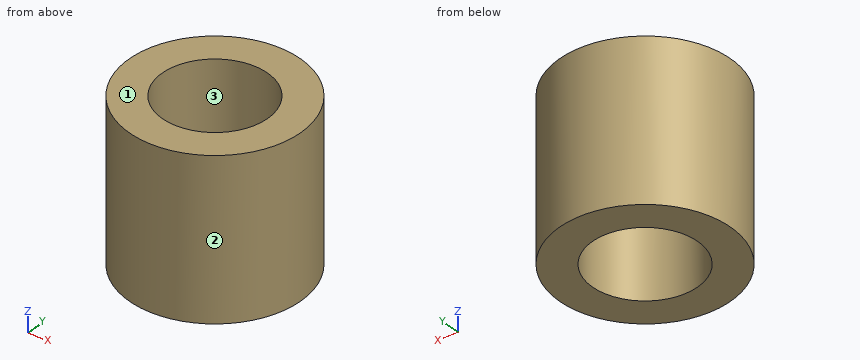
Autodesk Fusion 360 part; units mm, degrees
sketch "Sketch1" plane through (0, 0, 0) normal (0, 0, 1) x (1, 0, 0)
  circle A0 centre (0, 0) radius 2
  circle A1 centre (0, 0) radius 2.75
  dimension "d5" = 4
  dimension "d8" = 5.5
extrude "Extrude2" add sketch "Sketch1" along normal blind 6.6
move_face "OffsetFaces1" offset 0.5 1 faces at (2.7466, -0.1371, 4.4)
extrude "Extrude3" cut 1 faces at (2.8212, 0.1615, 6.6) along direction (0, 0, -1) blind 1.6
extrude "Extrude4" add 1 faces at (2.8212, 0.1615, 5) along direction (0, 0, 1) blind 1
Verification items for the finished model (mm, model axes). Face numbers are marked on the shaded views. Give positions to 0.01 mm unless a question says otherwise; leave off trailing zeros. Order: outer loops, then holes, each group sorted by start corner. A loop starts at its lowest first (then second) coordinate and runs counter-clockwise, first axis right, second up. Notation, with made-up numbers: M 4.25,75 L 47.25,75 A22 cw 47.25,95 Z; hole C 74,-32.5 d9. An arc over 180 degrees is marked long. Use one line per item in the form item = value. Start each with the question number.
Q1. Section check C-C (z = 0.6). Enter the section's corners in (x, y), then the cut area to 3 significant figures.
Q2. Go/stop test with a flat-tipped pin: pin 1 Ø3 at (x, z) = (2, 3.5) entering from +Y. Record where the tip stops, or that it passes through.
Q3. Section check A-A (x = 0). Enter the section's corners in (y, z), then the cut area to 3 significant figures.
Q4. Mould release check, pull along Y, two halves, no side actions. Record for the marked faces 1, 2 and 3: +Y half, -Y half, draft (parallel to the pull), parting line (faces both ways), or undercut.
Q5. Section check D-D (y = 3). Enter the section's corners in (x, z).
Q6. Scan lines: line 1 along Y through (x, z) = (0, 0.8); line 2 along Y through (x, z) = (-1.5, 0.6). Record each from-to range of solid material in increasing order. Write a range as [from, to].
Evaluation:
q1.outline = C 0,0 d6.5; hole C 0,0 d4
q1.area = 20.6 mm2
q2.pin_1 = 3.21
q3.outline = M -3.25,0 L -2,0 L -2,6 L -3.25,6 Z; M 2,0 L 3.25,0 L 3.25,6 L 2,6 Z
q3.area = 15.0 mm2
q4.face_1 = draft
q4.face_2 = parting line
q4.face_3 = undercut
q5.outline = M -1.25,0 L 1.25,0 L 1.25,6 L -1.25,6 Z
q6.line_1 = [-3.25, -2], [2, 3.25]
q6.line_2 = [-2.88, -1.32], [1.32, 2.88]
